```python
from build123d import *

# Parameters (mm, degrees)
SKETCH_1_W          = 340
SKETCH_1_H          = 240
EXTRUDE_1_DEPTH     = 10
FILLET_1_R          = 15
FILLET_2_R          = 15
FILLET_3_R          = 15
FILLET_4_R          = 15
SKETCH_2_R          = 5
CUT_EXTRUDE_1_DEPTH = 10


with BuildPart() as part:
    # 草图1 → 凸台-拉伸1 (new body)
    with BuildSketch(Plane.XY):
        Rectangle(SKETCH_1_W, SKETCH_1_H)
    extrude(amount=EXTRUDE_1_DEPTH)

    # 圆角1
    fillet_1_edges = [part.edges().sort_by_distance(p)[0] for p in [
        (-170, 120, 5),
    ]]
    fillet(fillet_1_edges, radius=FILLET_1_R)

    # 圆角2
    fillet_2_edges = [part.edges().sort_by_distance(p)[0] for p in [
        (170, 120, 5),
    ]]
    fillet(fillet_2_edges, radius=FILLET_2_R)

    # 圆角3
    fillet_3_edges = [part.edges().sort_by_distance(p)[0] for p in [
        (170, -120, 5),
    ]]
    fillet(fillet_3_edges, radius=FILLET_3_R)

    # 圆角4
    fillet_4_edges = [part.edges().sort_by_distance(p)[0] for p in [
        (-170, -120, 5),
    ]]
    fillet(fillet_4_edges, radius=FILLET_4_R)

    # 草图2 → 切除-拉伸1 (cut)
    with BuildSketch(Plane.XY.offset(10)):
        with Locations((110, 90)):
            Circle(SKETCH_2_R)
        with Locations((-110, 90)):
            Circle(SKETCH_2_R)
        with Locations(Location((110, -90, 0), (0, 0, 180))):
            Circle(SKETCH_2_R)
        with Locations(Location((-110, -90, 0), (0, 0, 180))):
            Circle(SKETCH_2_R)
    extrude(amount=-CUT_EXTRUDE_1_DEPTH, mode=Mode.SUBTRACT)


solid = part.part
```
CAD build for the part. Positions are in the model's coordinates, mm. Coordinates: 2 decimals unless noted, no trailing zeros. Write each loop counter-clockwise with the first axis right and the second up, starting at its lowest first coordinate (ties: lowest second). Pieces come first, ordered by that corner, then holes. Notation, with made-up numbers: (-13, 52.25) -> (18, 52.25) arc R16 cw to (18, 56.25) -> close; hole circle Ø1 at (55, 75). An arc over 180 degrees is marked (long way). Use CSV: the item, a comma, the result in double quotes. Start each with the question number.
Item 1: Band-saw the part on A-A, the plane x = -110. Write the cut outline in (y, z), plus the area to 3 significant figures.
Item 2: Wall check: probe 1 along X at (y, z) = (-90, 4.5); probe 2 along Y at (x, z) = (110, 3.75); probe 3 along Y at (x, z) = (-107, 5). Give the ranges that are in metal, low to high.
Item 3: Band-saw the part on B-B, the plane y = -90. Write the cut outline in (x, z), plus the area to 3 significant figures.
Item 4: Two-plate mould, pull along X, no slides. Class faces 1 (the cylindrical face through (165.49, 115.72, 5.07)), 2 (the flat face through (-2, -120, 5)), 3 (the cylindrical face through (105.381, -88.085, 5.07)): +X half, -X half, draft (parallel to the pull), parting line (faces both ways), or undercut.
Item 5: Drop flat-ended pins along their axis: P1, Ø6, axis at x = -52, y = 6.5, coming from the -Z side; P2, Ø8, axis at x = -110, y = 90, coming from the -Z side. Give the stop position or say it passes through.
Response values:
1,outline,"(-120, 0) -> (-95, 0) -> (-95, 10) -> (-120, 10) -> close; (-85, 0) -> (85, 0) -> (85, 10) -> (-85, 10) -> close; (95, 0) -> (120, 0) -> (120, 10) -> (95, 10) -> close"
1,area,"2,200 mm2"
2,probe 1,"x = -170 to -115, -105 to 105, 115 to 170"
2,probe 2,"y = -120 to -95, -85 to 85, 95 to 120"
2,probe 3,"y = -120 to -94, -86 to 86, 94 to 120"
3,outline,"(-170, 0) -> (-115, 0) -> (-115, 10) -> (-170, 10) -> close; (-105, 0) -> (105, 0) -> (105, 10) -> (-105, 10) -> close; (115, 0) -> (170, 0) -> (170, 10) -> (115, 10) -> close"
3,area,"3,200 mm2"
4,face 1,"+X half"
4,face 2,"draft"
4,face 3,"undercut"
5,P1,"stops at z = 0"
5,P2,"passes through"
